The listing builds one solid part. Answer for the finished solid, in the listing's coordinates (mm). Give positions to 0.01 mm unless a question says otherwise; leave off trailing zeros. Loops run counter-clockwise (first coordinate to the right, second up) from the corner with the lowest first, then second, coordinate; pieces in that order, holes last. Notation, with made-up numbers: M -6.75,-1.5 L 41.25,-1.5 A6 ccw 41.25,9.5 Z; hole C 60,-40 d8. An arc over 180 degrees is marked long. One line per item, written item: value. Start each with the question number.
Q1. A flat-ended cylindrical pin translates along its axis: pin 1 (5 mm diameter, centred on x = 224.24, y = 224.24, fed in from +Z). Find the tip coordinate at first contact, or state that the pin passes through.
Q2. A cutting plane is placed at B-B, the plane x = 25.4. Determine the outline of the cut face in (y, z).
Q3. A cutting plane is placed at D-D, the plane x = 108.5. Determine the outline of the cut face in (y, z).
Q4. The mould has two halves that part along X. Classify faces 1 (the cylindrical face through (283.066, 277.88, 0.783)), 2 (the flat face through (218, 87, 1.588)): +X half, -X half, draft (parallel to the pull), parting line (faces both ways), or undercut.
Q5. Consider L1, parallel to X at y = 221.5, z = 1.1; L2, parallel to Y at x = 50.8, z = 0.7; L3, parallel to X at y = 283, z = 1.4. Determine where each line is inside the solid, lowest interval first.
Q6. A cutting plane is placed at A-A, the plane y = 152.4. Determine the outline of the cut face in (x, z), and give its area (3 significant figures).
from build123d import *

# Parameters (mm, degrees)
F0_W     = 304.8
F0_H     = 304.8
F0_R     = 3.96875
F1_DEPTH = 1.5875
F2_R     = 88.9
F3_DEPTH = 25.4
F4_R     = 3.96875
F5_DEPTH = 25.4
F6_DEPTH = 25.4


with BuildPart() as f1:
    # F0 (on Top) → F1 (new body)
    with BuildSketch(Plane.XY):
        with Locations((152.4, 152.4)):
            Rectangle(F0_W, F0_H)
        with Locations((25.4, 25.4)):
            Circle(F0_R, mode=Mode.SUBTRACT)
        with Locations((279.4, 25.4)):
            Circle(F0_R, mode=Mode.SUBTRACT)
        with Locations((25.4, 279.4)):
            Circle(F0_R, mode=Mode.SUBTRACT)
        with Locations((279.4, 279.4)):
            Circle(F0_R, mode=Mode.SUBTRACT)
    extrude(amount=F1_DEPTH)

    # F2 (on face) → F3 (cut)
    with BuildSketch(Plane.XY.offset(1.5875)):
        with Locations((152.4, 152.4)):
            Circle(F2_R)
    extrude(amount=-F3_DEPTH, mode=Mode.SUBTRACT)

    # F4 (on face) → F5 (cut)
    with BuildSketch(Plane.XY.offset(1.5875)):
        with Locations((152.4, 254)):
            Circle(F4_R)
        with Locations((152.4, 50.8)):
            Circle(F4_R)
        with Locations((50.8, 152.4)):
            Circle(F4_R)
        with Locations((254, 152.4)):
            Circle(F4_R)
        with Locations((80.557951, 224.242049)):
            Circle(F4_R)
        with Locations((224.242049, 80.557951)):
            Circle(F4_R)
        with Locations((224.242049, 224.242049)):
            Circle(F4_R)
        with Locations((80.557951, 80.557951)):
            Circle(F4_R)
    extrude(amount=-F5_DEPTH, mode=Mode.SUBTRACT)

    # F4 (on face) → F6 (cut)
    with BuildSketch(Plane.XY.offset(1.5875)):
        with Locations((152.4, 254)):
            Circle(F4_R)
        with Locations((152.4, 50.8)):
            Circle(F4_R)
        with Locations((50.8, 152.4)):
            Circle(F4_R)
        with Locations((254, 152.4)):
            Circle(F4_R)
        with Locations((80.557951, 224.242049)):
            Circle(F4_R)
        with Locations((224.242049, 80.557951)):
            Circle(F4_R)
        with Locations((224.242049, 224.242049)):
            Circle(F4_R)
        with Locations((80.557951, 80.557951)):
            Circle(F4_R)
    extrude(amount=-F6_DEPTH, mode=Mode.SUBTRACT)


solid = f1.part
Answer block:
1. pin 1: through
2. outline: M 0,0 L 21.43,0 L 21.43,1.59 L 0,1.59 Z; M 29.37,0 L 275.43,0 L 275.43,1.59 L 29.37,1.59 Z; M 283.37,0 L 304.8,0 L 304.8,1.59 L 283.37,1.59 Z
3. outline: M 0,0 L 75.1,0 L 75.1,1.59 L 0,1.59 Z; M 229.7,0 L 304.8,0 L 304.8,1.59 L 229.7,1.59 Z
4. face 1: undercut
4. face 2: draft
5. L1: 0 to 77.69, 83.43 to 96.47, 208.33 to 221.37, 227.11 to 304.8
5. L2: 0 to 148.43, 156.37 to 304.8
5. L3: 0 to 23.73, 27.07 to 277.73, 281.07 to 304.8
6. outline: M 0,0 L 46.83,0 L 46.83,1.59 L 0,1.59 Z; M 54.77,0 L 63.5,0 L 63.5,1.59 L 54.77,1.59 Z; M 241.3,0 L 250.03,0 L 250.03,1.59 L 241.3,1.59 Z; M 257.97,0 L 304.8,0 L 304.8,1.59 L 257.97,1.59 Z
6. area: 176 mm^2
